Here's how the part is built. I have some questions about the finished solid (model axes, mm). Coordinates: 2 decimals unless noted, no trailing zeros. Write each loop counter-clockwise with the first axis right and the second up, starting at its lowest first coordinate (ties: lowest second). Pieces come first, ordered by that corner, then holes.
(1) Imagine slicing it at D-D, the plane z = 118. List the corners of the cut face in (x, y) for me.
(2) Imagine slicing it at B-B, the plane z = 225.5. List the corners of the cut face in (x, y) for me.
(3) For pin 1 Ø3 at (y, z) = (-4.5, 90) entering from -X; pin 2 Ø12 at (x, z) = (-77, 144) entering from +Y; pin 3 Ø3 at (y, z) = (-3, 228.5) entering from -X; pin 4 Ø5 at (y, z) = (-4.5, 281.5) entering from -X, each with a flat end and sliding along its axis, tell me the tip position at first contact or that it passes through.
(4) Please list where these lines run through material, in increasing order: probe 1 along Z at (x, y) = (-264.5, -9); probe 2 along X at (y, z) = (-2.25, 155); probe 3 along X at (y, z) = (-9.25, -98).
(5) Imagine slicing it at C-C, the plane x = 174. List the corners of the cut face in (y, z) for me, plus the area to 3 significant figures.
(6) Imagine slicing it at A-A, the plane x = 0. List the corners of the cut face in (y, z) for me.
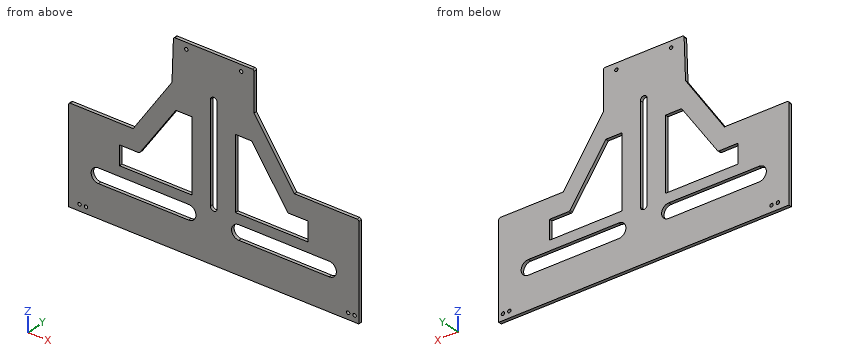
```python
from build123d import *

# Parameters (mm, degrees)
F0_R     = 5.25
F1_DEPTH = 10
F2_R     = 5
F3_R     = 5


# Not quite as in the source:
# - ends of sketch curves that miss each other by under 0.0002 mm in the source are joined


with BuildPart() as f1:
    # F0 (on Front) → F1 (new body)
    with BuildSketch(Plane.XZ):
        Polygon((-250, 62.7604842186), (-450, 62.7604842186), (-450, -237.2395157814), (0, -237.2395157814), (450, -237.2395157814), (450, 62.7604842186), (250, 62.7604842186), (125, 247.7604842186), (125, 372.7604842186), (-125, 372.7604842186), (-129.5981111256, 240.9552797528), align=None)
        with Locations((-416.2039160728, -217.2395157814)):
            Circle(F0_R, mode=Mode.SUBTRACT)
        with Locations((-396.2039160728, -217.2395157814)):
            Circle(F0_R, mode=Mode.SUBTRACT)
        with BuildLine():
            Line((-357.8152358532, -90.9260827303), (-77.8152358532, -90.9260827303))
            ThreePointArc((-77.8152358532, -90.9260827303), (-55.3152358532, -113.4260827303), (-77.8152358532, -135.9260827303))
            Line((-77.8152358532, -135.9260827303), (-357.8152358532, -135.9260827303))
            ThreePointArc((-357.8152358532, -135.9260827303), (-380.3152358532, -113.4260827303), (-357.8152358532, -90.9260827303))
        make_face(mode=Mode.SUBTRACT)
        Polygon((-292.343990892, -60), (-292.343990892, 0), (-230.3705364466, 0), (-117.343990892, 165), (-67.343990892, 165), (-67.343990892, 0), (-67.343990892, -60), align=None, mode=Mode.SUBTRACT)
        with BuildLine():
            ThreePointArc((77.8152358532, -135.9260827303), (55.3152358532, -113.4260827303), (77.8152358532, -90.9260827303))
            Line((77.8152358532, -90.9260827303), (357.8152358532, -90.9260827303))
            ThreePointArc((357.8152358532, -90.9260827303), (380.3152358532, -113.4260827303), (357.8152358532, -135.9260827303))
            Line((357.8152358532, -135.9260827303), (77.8152358532, -135.9260827303))
        make_face(mode=Mode.SUBTRACT)
        with Locations((416.8414473534, -217.2395157814)):
            Circle(F0_R, mode=Mode.SUBTRACT)
        with Locations((436.8414473534, -217.2395157814)):
            Circle(F0_R, mode=Mode.SUBTRACT)
        Polygon((67.343990892, 0), (67.343990892, 165), (117.343990892, 165), (230.3705364466, 0), (292.343990892, 0), (292.343990892, -60), (67.343990892, -60), align=None, mode=Mode.SUBTRACT)
        with Locations((-85, 352.7604842186)):
            Circle(F0_R, mode=Mode.SUBTRACT)
        with BuildLine():
            Line((-10.5, 235.874648428), (-10.5, 235.897347331))
            ThreePointArc((-10.5, 235.897347331), (0.0113494317, 246.3746422942), (10.5, 235.874648428))
            Line((10.5, 235.874648428), (10.5, 0.0226989031))
            Line((10.5, 0.0226989031), (10.5, -70.725351572))
            ThreePointArc((10.5, -70.725351572), (0, -81.225351572), (-10.5, -70.725351572))
            Line((-10.5, -70.725351572), (-10.5, 0))
            Line((-10.5, 0), (-10.5, 235.874648428))
        make_face(mode=Mode.SUBTRACT)
        with Locations((85, 352.7604842186)):
            Circle(F0_R, mode=Mode.SUBTRACT)
    extrude(amount=F1_DEPTH)

    # F2
    f2_edges = [f1.edges().sort_by_distance(p)[0] for p in [
        (-230.370536, -5, 0),
        (230.370536, -5, 0),
    ]]
    fillet(f2_edges, radius=F2_R)

    # F3
    f3_edges = [f1.edges().sort_by_distance(p)[0] for p in [
        (-450, -5, 62.760484),
        (-125, -5, 372.760484),
        (125, -5, 372.760484),
        (450, -5, 62.760484),
    ]]
    fillet(f3_edges, radius=F3_R)


solid = f1.part
```
Recorded:
1. outline: (-212.68, -10) - (-149.54, -10) - (-149.54, 0) - (-212.68, 0) - close; (-67.34, -10) - (-10.5, -10) - (-10.5, 0) - (-67.34, 0) - close; (10.5, -10) - (67.34, -10) - (67.34, 0) - (10.5, 0) - close; (149.54, -10) - (212.68, -10) - (212.68, 0) - (149.54, 0) - close
2. outline: (-140.04, -10) - (-10.5, -10) - (-10.5, 0) - (-140.04, 0) - close; (10.5, -10) - (140.04, -10) - (140.04, 0) - (10.5, 0) - close
3. pin 1: stops at x = -232.61
3. pin 2: passes through
3. pin 3: stops at x = -139.03
3. pin 4: stops at x = -128.27
4. probe 1: z = -237.24 to -135.93, -90.93 to -60, 0 to 62.76
4. probe 2: x = -187.68 to -124.19, -67.34 to -10.5, 10.5 to 67.34, 124.19 to 187.68
4. probe 3: x = -450 to -374.19, -61.44 to 61.44, 374.19 to 450
5. outline: (-10, -237.24) - (0, -237.24) - (0, -135.93) - (-10, -135.93) - close; (-10, -90.93) - (0, -90.93) - (0, -60) - (-10, -60) - close; (-10, 82.29) - (0, 82.29) - (0, 175.24) - (-10, 175.24) - close
5. area: 2,250 mm2
6. outline: (-10, -237.24) - (0, -237.24) - (0, -81.23) - (-10, -81.23) - close; (-10, 246.37) - (0, 246.37) - (0, 372.76) - (-10, 372.76) - close
